CAD build for the part. Positions are in the model's coordinates, mm. A direction names the side the tool comes from. Round coordinates to 2 decimals unless told otherwise and drop trailing zeros. Loops run counter-clockwise (first coordinate to the right, second up) from the corner with the lowest first, then second, coordinate; pieces in that order, holes last.
from build123d import *

# Parameters (mm, degrees)
SKETCH_1_W            = 36
SKETCH_1_H            = 40
EXTRUDE_1_DEPTH       = 3
SKETCH_2_W            = 3
SKETCH_2_H            = 40
EXTRUDE_2_DEPTH       = 18.8
SKETCH_3_R            = 14
CUT_EXTRUDE_1_DEPTH   = 9
SKETCH_4_W            = 36
SKETCH_4_H            = 3
EXTRUDE_3_DEPTH       = 10
SKETCH_6_R            = 2.7
CUT_EXTRUDE_3_DEPTH   = 10
SKETCH_7_R            = 1.75
CUT_EXTRUDE_4_DEPTH   = 52.68404009
SKETCH_9_W            = 25
SKETCH_9_H            = 3
SKETCH_9_W_2          = 3
SKETCH_9_H_2          = 9.3
EXTRUDE_4_DEPTH       = 20
CHAMFER_1_SIZE        = 5
CUT_EXTRUDE_START     = -30
SKETCH_10_R           = 2.7
CUT_EXTRUDE_5_DEPTH   = 30
SKETCH_11_W           = 40.05397725
SKETCH_11_H           = 18.071111192
CUT_EXTRUDE_6_DEPTH   = 52.68404009
EXTRUDE_START         = 2.5
SKETCH_12_W           = 36
SKETCH_12_H           = 20
SKETCH_12_R           = 2.7
EXTRUDE_5_DEPTH       = 2.5
SKETCH_13_W           = 62.12277329
SKETCH_13_H           = 35.561448302
CUT_EXTRUDE_7_DEPTH   = 1
SKETCH_16_W           = 60
SKETCH_16_H           = 3
SKETCH_16_W_2         = 3
SKETCH_16_H_2         = 25
EXTRUDE_7_DEPTH       = 65
EXTRUDE_START_2       = 8
EXTRUDE_8_DEPTH       = 8
SKETCH_18_R           = 1.15
SKETCH_18_R_2         = 10
CUT_EXTRUDE_8_DEPTH   = 15
SKETCH_19_W           = 125.229267156
SKETCH_19_H           = 103.922898786
CUT_EXTRUDE_9_DEPTH   = 0.5
SKETCH_20_W           = 154.797288569
SKETCH_20_H           = 90.443359613
CUT_EXTRUDE_10_DEPTH  = 1.8
SKETCH_21_W           = 11.155684717
SKETCH_21_H           = 2.603751016
EXTRUDE_9_DEPTH       = 3
EXTRUDE_10_DEPTH      = 10
EXTRUDE_10_DEPTH_BACK = 4
SKETCH_22_W           = 36
SKETCH_22_H           = 3.2
SKETCH_23_R           = 1.75
CUT_EXTRUDE_12_DEPTH  = 10
SKETCH_26_W           = 12.845915964
SKETCH_26_H           = 7.377373426
EXTRUDE_11_DEPTH      = 3.2
SKETCH_27_W           = 116.42408431
SKETCH_27_H           = 62.505927617
CUT_EXTRUDE_13_DEPTH  = 10
SKETCH_29_W           = 89.791123847
SKETCH_29_H           = 12.28472202
SKETCH_29_W_2         = 107.401489541
SKETCH_29_H_2         = 29.785433334
CUT_EXTRUDE_14_DEPTH  = 25
SKETCH_30_W           = 3
SKETCH_30_H           = 18.8
EXTRUDE_12_DEPTH      = 17
SKETCH_31_W           = 80.768529078
SKETCH_31_H           = 45.765209612
CUT_EXTRUDE_15_DEPTH  = 0.6
SKETCH_32_W           = 23
SKETCH_32_H           = 2.8
SKETCH_32_W_2         = 3
SKETCH_32_H_2         = 9.9
EXTRUDE_13_DEPTH      = 14
SKETCH_34_R           = 1.75
CUT_EXTRUDE_17_DEPTH  = 97.806198149
SKETCH_35_W           = 168.711651586
SKETCH_35_H           = 128.925269833
CUT_EXTRUDE_18_DEPTH  = 7
SKETCH_36_W           = 30.780953922
SKETCH_36_H           = 20.383466973
CUT_EXTRUDE_19_DEPTH  = 43.8


with BuildPart() as part:
    # 草图1 → 凸台-拉伸1 (new body)
    with BuildSketch(Plane(origin=(0, 0, 0), x_dir=(1, 0, 0), z_dir=(0, 1, 0))):
        Rectangle(SKETCH_1_W, SKETCH_1_H)
    extrude(amount=EXTRUDE_1_DEPTH)

    # 草图2 → 凸台-拉伸2 (add)
    with BuildSketch(Plane(origin=(0, 3, 0), x_dir=(1, 0, 0), z_dir=(0, 1, 0))):
        with Locations((-16.5, 0)):
            Rectangle(SKETCH_2_W, SKETCH_2_H)
        with Locations((16.5, 0)):
            Rectangle(SKETCH_2_W, SKETCH_2_H)
    extrude(amount=EXTRUDE_2_DEPTH)

    # 草图3 → 切除-拉伸1 (cut)
    with BuildSketch(Plane(origin=(0, 0, 0), x_dir=(-1, 0, 0), z_dir=(0, -1, 0))):
        with Locations(Location((-2.75, 3.000025, 0), (0, 0, 90))):
            Circle(SKETCH_3_R)
    extrude(amount=-CUT_EXTRUDE_1_DEPTH, mode=Mode.SUBTRACT)

    # 草图4 → 凸台-拉伸3 (add)
    with BuildSketch(Plane.XY.offset(20)):
        with Locations((0, 1.5)):
            Rectangle(SKETCH_4_W, SKETCH_4_H)
    extrude(amount=EXTRUDE_3_DEPTH)

    # 草图6 → 切除-拉伸3 (cut)
    with BuildSketch(Plane(origin=(0, 0, 0), x_dir=(-1, 0, 0), z_dir=(0, -1, 0))):
        with Locations(Location((-2.75, -16.149975, 0), (0, 0, 90))):
            Circle(SKETCH_6_R)
    extrude(amount=-CUT_EXTRUDE_3_DEPTH, mode=Mode.SUBTRACT)

    # 草图7 → 切除-拉伸4 (cut, through all)
    with BuildSketch(Plane.ZY.offset(18)):
        with Locations((15, 18.8)):
            Circle(SKETCH_7_R)
        with Locations((-5, 18.8)):
            Circle(SKETCH_7_R)
    extrude(amount=-CUT_EXTRUDE_4_DEPTH, mode=Mode.SUBTRACT)

    # 草图9 → 凸台-拉伸4 (add)
    with BuildSketch(Plane.XY.offset(30)):
        with Locations((-2.5, -7.8)):
            Rectangle(SKETCH_9_W, SKETCH_9_H)
        with Locations((-16.5, -4.65)):
            Rectangle(SKETCH_9_W_2, SKETCH_9_H_2)
    extrude(amount=-EXTRUDE_4_DEPTH)

    # 倒角1
    chamfer_1_edges = [part.edges().sort_by_distance(p)[0] for p in [
        (10, -7.8, 30),
    ]]
    chamfer(chamfer_1_edges, length=CHAMFER_1_SIZE)

    # 草图10 → 切除-拉伸5 (cut)
    with BuildSketch(Plane(origin=(0, 0, 0), x_dir=(1, 0, 0), z_dir=(0, 1, 0)).offset(CUT_EXTRUDE_START)):
        with Locations(Location((2.75, -16.149975, 0), (0, 0, 90))):
            Circle(SKETCH_10_R)
    extrude(amount=CUT_EXTRUDE_5_DEPTH, mode=Mode.SUBTRACT)

    # 草图11 → 切除-拉伸6 (cut, through all)
    with BuildSketch(Plane.ZY.offset(18)):
        with Locations((20.026988625, -9.035555596)):
            Rectangle(SKETCH_11_W, SKETCH_11_H)
    extrude(amount=-CUT_EXTRUDE_6_DEPTH, mode=Mode.SUBTRACT)

    # 草图12 → 凸台-拉伸5 (add)
    with BuildSketch(Plane(origin=(0, 0, 0), x_dir=(-1, 0, 0), z_dir=(0, -1, 0)).offset(EXTRUDE_START)):
        with Locations((0, -20)):
            Rectangle(SKETCH_12_W, SKETCH_12_H)
        with Locations(Location((-2.75, -16.149975, 0), (0, 0, 90))):
            Circle(SKETCH_12_R, mode=Mode.SUBTRACT)
    extrude(amount=-EXTRUDE_5_DEPTH)

    # 草图13 → 切除-拉伸7 (cut)
    with BuildSketch(Plane(origin=(0, 0, 0), x_dir=(-1, 0, 0), z_dir=(0, -1, 0))):
        with Locations((0.086945799, 7.780724151)):
            Rectangle(SKETCH_13_W, SKETCH_13_H)
    extrude(amount=-CUT_EXTRUDE_7_DEPTH, mode=Mode.SUBTRACT)

    # 草图16 → 凸台-拉伸7 (add)
    with BuildSketch(Plane.XY.offset(20)):
        with Locations((48, 45.3)):
            Rectangle(SKETCH_16_W, SKETCH_16_H)
        with Locations((16.5, 34.3)):
            Rectangle(SKETCH_16_W_2, SKETCH_16_H_2)
    extrude(amount=-EXTRUDE_7_DEPTH)

    # 草图17 → 凸台-拉伸8 (add)
    with BuildSketch(Plane(origin=(0, 9, 0), x_dir=(-1, 0, 0), z_dir=(0, -1, 0)).offset(EXTRUDE_START_2)):
        with BuildLine():
            Line((-15, -3.777695856), (-15, 9.777745856))
            ThreePointArc((-15, 9.777745856), (-16.75, 3.000025), (-15, -3.777695856))
        make_face()
    extrude(amount=-EXTRUDE_8_DEPTH)

    # 草图18 → 切除-拉伸8 (cut)
    with BuildSketch(Plane(origin=(0, 46.8, 0), x_dir=(1, 0, 0), z_dir=(0, 1, 0))):
        with Locations(Location((47.75, 25.75, 0), (0, 0, 270))):
            Circle(SKETCH_18_R)
        with Locations(Location((74.25, 25.75, 0), (0, 0, 270))):
            Circle(SKETCH_18_R)
        with Locations(Location((74.25, -0.75, 0), (0, 0, 270))):
            Circle(SKETCH_18_R)
        with Locations(Location((47.75, -0.75, 0), (0, 0, 270))):
            Circle(SKETCH_18_R)
        with Locations(Location((61, 12.5, 0), (0, 0, 270))):
            Circle(SKETCH_18_R_2)
        with BuildLine():
            Line((52, 27.75), (70, 27.75))
            ThreePointArc((70, 27.75), (72, 25.75), (70, 23.75))
            Line((70, 23.75), (52, 23.75))
            ThreePointArc((52, 23.75), (50, 25.75), (52, 27.75))
        make_face()
        with BuildLine():
            Line((52, -2.75), (70, -2.75))
            ThreePointArc((70, -2.75), (72, -0.75), (70, 1.25))
            Line((70, 1.25), (52, 1.25))
            ThreePointArc((52, 1.25), (50, -0.75), (52, -2.75))
        make_face()
    extrude(amount=-CUT_EXTRUDE_8_DEPTH, mode=Mode.SUBTRACT)

    # 草图19 → 切除-拉伸9 (cut)
    with BuildSketch(Plane(origin=(0, -2.5, 0), x_dir=(-1, 0, 0), z_dir=(0, -1, 0))):
        with Locations((5.272239112, -16.1971882)):
            Rectangle(SKETCH_19_W, SKETCH_19_H)
    extrude(amount=-CUT_EXTRUDE_9_DEPTH, mode=Mode.SUBTRACT)

    # 草图20 → 切除-拉伸10 (cut)
    with BuildSketch(Plane(origin=(0, -2, 0), x_dir=(-1, 0, 0), z_dir=(0, -1, 0))):
        with Locations((2.880707968, -7.718123237)):
            Rectangle(SKETCH_20_W, SKETCH_20_H)
    extrude(amount=-CUT_EXTRUDE_10_DEPTH, mode=Mode.SUBTRACT)

    # 草图21 → 凸台-拉伸9 (add)
    with BuildSketch(Plane(origin=(0, 0, 0), x_dir=(1, 0, 0), z_dir=(0, 1, 0))):
        with Locations((3.131752483, -11.301875508)):
            Rectangle(SKETCH_21_W, SKETCH_21_H)
    extrude(amount=EXTRUDE_9_DEPTH)

    # 草图22 → 凸台-拉伸10 (add, two sides: drawn at the far end of the back side and taken through both)
    with BuildSketch(Plane(origin=(0, 0, -20), x_dir=(-1, 0, 0), z_dir=(0, 0, -1)).offset(-EXTRUDE_10_DEPTH_BACK)):
        with Locations((0, 1.4)):
            Rectangle(SKETCH_22_W, SKETCH_22_H)
    extrude(amount=EXTRUDE_10_DEPTH + EXTRUDE_10_DEPTH_BACK)

    # 草图23 → 切除-拉伸12 (cut)
    with BuildSketch(Plane(origin=(0, 9, 0), x_dir=(-1, 0, 0), z_dir=(0, -1, 0))):
        with Locations(Location((-2.75, 22.150025, 0), (0, 0, 270))):
            Circle(SKETCH_23_R)
    extrude(amount=CUT_EXTRUDE_12_DEPTH, mode=Mode.SUBTRACT)

    # 草图26 → 凸台-拉伸11 (add, through all)
    with BuildSketch(Plane(origin=(0, 3, 0), x_dir=(1, 0, 0), z_dir=(0, 1, 0))):
        with Locations((3.420651678, -16.929062366)):
            Rectangle(SKETCH_26_W, SKETCH_26_H)
    extrude(amount=-EXTRUDE_11_DEPTH)

    # 草图27 → 切除-拉伸13 (cut)
    with BuildSketch(Plane.XY.offset(30)):
        with Locations((4.783062287, -2.648783639)):
            Rectangle(SKETCH_27_W, SKETCH_27_H)
    extrude(amount=-CUT_EXTRUDE_13_DEPTH, mode=Mode.SUBTRACT)

    # 草图29 → 切除-拉伸14 (cut)
    with BuildSketch(Plane(origin=(0, 46.8, 0), x_dir=(1, 0, 0), z_dir=(0, 1, 0))):
        with Locations((43.319325488, 43.14236101)):
            Rectangle(SKETCH_29_W, SKETCH_29_H)
        with Locations((56.472746777, -26.892716667)):
            Rectangle(SKETCH_29_W_2, SKETCH_29_H_2)
    extrude(amount=-CUT_EXTRUDE_14_DEPTH, mode=Mode.SUBTRACT)

    # 草图30 → 凸台-拉伸12 (add)
    with BuildSketch(Plane(origin=(0, 0, -20), x_dir=(-1, 0, 0), z_dir=(0, 0, -1))):
        with Locations((-16.5, 12.4)):
            Rectangle(SKETCH_30_W, SKETCH_30_H)
    extrude(amount=EXTRUDE_12_DEPTH)

    # 草图31 → 切除-拉伸15 (cut)
    with BuildSketch(Plane(origin=(0, -0.2, 0), x_dir=(-1, 0, 0), z_dir=(0, -1, 0))):
        with Locations((-3.369884793, 29.731080354)):
            Rectangle(SKETCH_31_W, SKETCH_31_H)
    extrude(amount=-CUT_EXTRUDE_15_DEPTH, mode=Mode.SUBTRACT)

    # 草图32 → 凸台-拉伸13 (add)
    with BuildSketch(Plane(origin=(0, 0, -30), x_dir=(-1, 0, 0), z_dir=(0, 0, -1))):
        with Locations((3.5, -8.3)):
            Rectangle(SKETCH_32_W, SKETCH_32_H)
        with Locations((16.5, -1.95)):
            Rectangle(SKETCH_32_W_2, SKETCH_32_H_2)
        with Locations((16.5, -8.3)):
            Rectangle(SKETCH_32_W_2, SKETCH_32_H)
    extrude(amount=-EXTRUDE_13_DEPTH)

    # 草图34 → 切除-拉伸17 (cut, through all)
    with BuildSketch(Plane(origin=(0, 3, 0), x_dir=(1, 0, 0), z_dir=(0, 1, 0))):
        with Locations(Location((2.75, 22.150025, 0), (0, 0, 270))):
            Circle(SKETCH_34_R)
    extrude(amount=-CUT_EXTRUDE_17_DEPTH, mode=Mode.SUBTRACT)

    # 草图35 → 切除-拉伸18 (cut)
    with BuildSketch(Plane(origin=(0, 0, -37), x_dir=(-1, 0, 0), z_dir=(0, 0, -1))):
        with Locations((-14.403539842, 2.608943066)):
            Rectangle(SKETCH_35_W, SKETCH_35_H)
    extrude(amount=-CUT_EXTRUDE_18_DEPTH, mode=Mode.SUBTRACT)

    # 草图36 → 切除-拉伸19 (cut)
    with BuildSketch(Plane(origin=(0, 46.8, 0), x_dir=(1, 0, 0), z_dir=(0, 1, 0))):
        with Locations((25.609523039, 30.191733487)):
            Rectangle(SKETCH_36_W, SKETCH_36_H)
    extrude(amount=-CUT_EXTRUDE_19_DEPTH, mode=Mode.SUBTRACT)


solid = part.part
Item 1: Mould opens along Z. For faces 1 (the cylindrical face through (52.128, 45.321, -7.886)), 2 (the flat face through (8, -8, -23)), 3 (the flat face through (17, 31, -20)) say: released by +Z, released by -Z, zero draft, split by the parting line, or undercut.
Verdict:
face 1: undercut
face 2: zero draft
face 3: released by -Z
Item 2: Cut at C-C (z = -25.75). List the corners of the cut face in (x, y).
Verdict:
outline: (-18, -9.7) - (8, -9.7) - (8, -6.9) - (-15, -6.9) - (-15, 0.4) - (18, 0.4) - (18, 3) - (-18, 3) - close; (41, 43.8) - (46.6, 43.8) - (46.6, 46.8) - (41, 46.8) - close; (48.9, 43.8) - (50, 43.8) - (50, 46.8) - (48.9, 46.8) - close; (72, 43.8) - (73.1, 43.8) - (73.1, 46.8) - (72, 46.8) - close; (75.4, 43.8) - (78, 43.8) - (78, 46.8) - (75.4, 46.8) - close
Item 3: Cut at B-B (y = 18.8). List the corners of the cut face in (x, z).
Verdict:
outline: (-18, -20) - (-15, -20) - (-15, -6.75) - (-18, -6.75) - close; (-18, -3.25) - (-15, -3.25) - (-15, 13.25) - (-18, 13.25) - close; (-18, 16.75) - (-15, 16.75) - (-15, 20) - (-18, 20) - close; (15, -20) - (18, -20) - (18, -6.75) - (15, -6.75) - close; (15, -3.25) - (18, -3.25) - (18, 13.25) - (15, 13.25) - close; (15, 16.75) - (18, 16.75) - (18, 20) - (15, 20) - close
Item 4: 3-axis set-ups, long thin cutter, end or side, ignore diameter. For faces 4 (the flat face through (2, 0.4, -25)), 5 (the flat face through (-3, -6.9, -23)), 6 (the flat face through (61, 45, -23.75)), 7 (the flat face through (0, 1, 10)): which of +Z, -Z, +X, -X, +Y, -Y reach the whole face in a straight line?
Verdict:
face 4: -Z, +X
face 5: +Z, -Z, +X
face 6: +Y, -Y
face 7: -Y
Item 5: Wall check: L1, parallel to Y at x = 3, z = -19; L2, parallel to Y at x = 16, z = -5; L3, parallel to Z at x = 74.25, y = 44.8. Give the ranges that are in metal, low to high.
Verdict:
L1: y = -9.7 to -6.9, 0.4 to 3
L2: y = 1 to 17.05, 20.55 to 46.8
L3: z = -30 to -26.9, -24.6 to -0.4, 1.9 to 12
Item 6: Cut at A-A (x = 47.75). List the corners of the cut face in (y, z), plus the area to 3 significant figures.
Verdict:
outline: (43.8, -30) - (46.8, -30) - (46.8, -26.9) - (43.8, -26.9) - close; (43.8, -24.6) - (46.8, -24.6) - (46.8, -0.4) - (43.8, -0.4) - close; (43.8, 1.9) - (46.8, 1.9) - (46.8, 12) - (43.8, 12) - close
area: 112 mm2
Item 7: Flat gauge pins, fed straight in: P1, Ø3, axis at x = 2.75, z = -22.15, coming from the +Y side; P2, Ø20, axis at y = 33, z = 6.5, coming from the -X side; P3, Ø2, axis at y = -3.5, z = -20, coming from the +X side; P4, Ø4, axis at x = 11, z = -15.5, coming from the -Y side. Where does each tip first touch, or does it go through?
Verdict:
P1: passes through
P2: stops at x = 15
P3: stops at x = -15
P4: stops at y = 0.4
Item 8: Cut at D-D (x = 61). List the corners of the cut face in (y, z), plus the area to 3 significant figures.
Verdict:
outline: (43.8, -30) - (46.8, -30) - (46.8, -27.75) - (43.8, -27.75) - close; (43.8, -23.75) - (46.8, -23.75) - (46.8, -22.5) - (43.8, -22.5) - close; (43.8, -2.5) - (46.8, -2.5) - (46.8, -1.25) - (43.8, -1.25) - close; (43.8, 2.75) - (46.8, 2.75) - (46.8, 12) - (43.8, 12) - close
area: 42.0 mm2
